Model file for the job. Use its own axes, mm. Face numbers are marked on the shaded views. Give positions to 0.01 mm unless a question says otherwise; leave off trailing zeros. Write each loop counter-clockwise with the first axis right and the second up, starting at its lowest first coordinate (ties: lowest second). Pieces come first, ordered by that corner, then holes. Notation, with made-up numbers: (-15.5, 10.25) - (15.5, 10.25) arc R24 cw to (15.5, 40.25) - close; hole circle Ø3 at (51, -34). An arc over 180 degrees is marked (long way). One line per item, written item: value. Start each with the question number.
(1) Drop flat-ended pins along their axis: P1, Ø3, axis at x = 0, z = 7, coming from the +Y side; P2, Ø4, axis at x = 0, z = -7, coming from the -Y side. Give the stop position or say it passes through.
(2) Cut at B-B, the plane y = 1.55. List the corners of the cut face in (x, z).
(3) Cut at D-D, the plane z = -7.5. List the corners of the cut face in (x, y), and give its area (3 significant figures).
(4) Probe L1, parallel to X at y = 1.6, z = -27.5; L2, parallel to Z at x = -3.25, y = 2.85; L3, parallel to Z at x = 2.25, y = 1.25. List the from-to ranges inside material, lowest first.
(5) Cut at A-A, the plane x = 0. List the corners of the cut face in (y, z).
(6) Cut at C-C, the plane x = 8. List the corners of the cut face in (y, z).
(7) Mould opens along Z. For the marked faces 1, 2, 3 and 4 say: pulls with the +Z half, pulls with the -Z half, needs draft (parallel to the pull), parting line crosses it, or undercut.
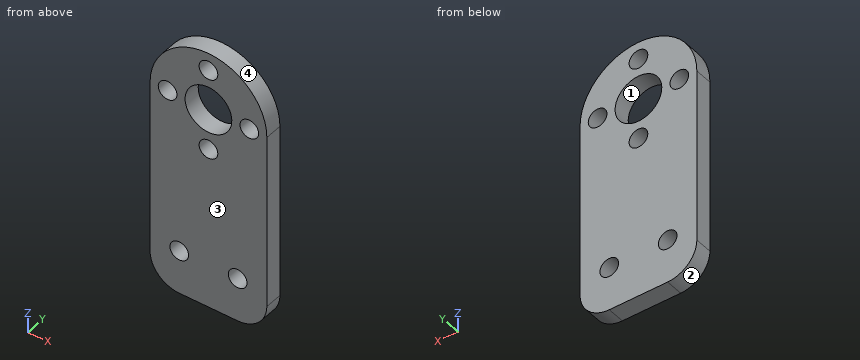
from build123d import *

# Parameters (mm, degrees)
SKETCH_1_R      = 1.6
SKETCH_1_R_2    = 4
EXTRUDE_1_DEPTH = 3
FILLET_1_R      = 5


with BuildPart() as part:
    # 草图1 → 凸台-拉伸1 (new body)
    with BuildSketch(Plane(origin=(0, 0, 0), x_dir=(1, 0, 0), z_dir=(0, 1, 0))):
        with BuildLine():
            Line((-10, 0), (-10, 35))
            Line((-10, 35), (10, 35))
            Line((10, 35), (10, 0))
            ThreePointArc((10, 0), (0, -10), (-10, 0))
        make_face()
        with Locations(Location((-5, 27.5, 0), (0, 0, 270))):
            Circle(SKETCH_1_R, mode=Mode.SUBTRACT)
        with Locations(Location((5, 27.5, 0), (0, 0, 270))):
            Circle(SKETCH_1_R, mode=Mode.SUBTRACT)
        with Locations(Location((0, 7, 0), (0, 0, 270))):
            Circle(SKETCH_1_R, mode=Mode.SUBTRACT)
        with Locations(Location((-7, 0, 0), (0, 0, 270))):
            Circle(SKETCH_1_R, mode=Mode.SUBTRACT)
        with Locations(Location((0, -7, 0), (0, 0, 270))):
            Circle(SKETCH_1_R, mode=Mode.SUBTRACT)
        with Locations(Location((7, 0, 0), (0, 0, 270))):
            Circle(SKETCH_1_R, mode=Mode.SUBTRACT)
        with Locations(Location((0, 0, 0), (0, 0, 270))):
            Circle(SKETCH_1_R_2, mode=Mode.SUBTRACT)
    extrude(amount=EXTRUDE_1_DEPTH)

    # 圆角1
    fillet_1_edges = [part.edges().sort_by_distance(p)[0] for p in [
        (-10, 1.5, -35),
        (10, 1.5, -35),
    ]]
    fillet(fillet_1_edges, radius=FILLET_1_R)


solid = part.part
Answers follow:
1. P1: passes through
1. P2: stops at y = 0
2. outline: (-10, -30) arc R5 ccw to (-5, -35) - (5, -35) arc R5 ccw to (10, -30) - (10, 0) arc R10 ccw to (-10, 0) - close; hole circle Ø3.2 at (-7, 0); hole circle Ø3.2 at (-5, -27.5); hole circle Ø8 at (0, 0); hole circle Ø3.2 at (0, -7); hole circle Ø3.2 at (0, 7); hole circle Ø3.2 at (5, -27.5); hole circle Ø3.2 at (7, 0)
3. outline: (-10, 0) - (-1.52, 0) - (-1.52, 3) - (-10, 3) - close; (1.52, 0) - (10, 0) - (10, 3) - (1.52, 3) - close
3. area: 50.9 mm²
4. L1: x = -10 to -6.6, -3.4 to 3.4, 6.6 to 10
4. L2: z = -35 to -2.33, 2.33 to 9.46
4. L3: z = -35 to -3.31, 3.31 to 9.74
5. outline: (0, -35) - (3, -35) - (3, -8.6) - (0, -8.6) - close; (0, -5.4) - (3, -5.4) - (3, -4) - (0, -4) - close; (0, 4) - (3, 4) - (3, 5.4) - (0, 5.4) - close; (0, 8.6) - (3, 8.6) - (3, 10) - (0, 10) - close
6. outline: (0, -34) - (3, -34) - (3, -1.25) - (0, -1.25) - close; (0, 1.25) - (3, 1.25) - (3, 6) - (0, 6) - close
7. face 1: undercut
7. face 2: pulls with the -Z half
7. face 3: needs draft
7. face 4: pulls with the +Z half
